For this review, take the finished solid that the model builds, in its own axes (mm). A direction names the side the tool comes from. Coordinates: 2 decimals unless noted, no trailing zeros. Loops run counter-clockwise (first coordinate to the right, second up) from the corner with the lowest first, then second, coordinate; pieces in that order, holes last. Notation, with made-up numbers: (-26.5, 80.25) -> (-14.5, 80.25) arc R3 cw to (-14.5, 84.25) -> close; hole circle Ø7 at (80.25, 86.25). An arc over 180 degrees is marked (long way). Use a Markdown table: item, result.
from build123d import *

# Parameters (mm, degrees)
SKETCH1_R           = 10.16
BOSS_EXTRUDE1_DEPTH = 88.9
FILLET1_R           = 2.54
SKETCH3_W           = 15.24
SKETCH3_H           = 10.16
BOSS_EXTRUDE2_DEPTH = 30.48
FILLET2_R           = 7.62
CUT_EXTRUDE1_REACH  = 97.208
SKETCH4_R           = 5.08
FILLET3_R           = 2.54


with BuildPart() as part:
    # Sketch1 → Boss-Extrude1 (new, symmetric)
    with BuildSketch(Plane.XY):
        Circle(SKETCH1_R)
    extrude(amount=BOSS_EXTRUDE1_DEPTH, both=True)

    # Fillet1
    fillet1_edges = [part.edges().sort_by_distance(p)[0] for p in [
        (-10.16, 0, -88.9),
        (-10.16, 0, 88.9),
    ]]
    fillet(fillet1_edges, radius=FILLET1_R)

    # Sketch3 → Boss-Extrude2 (add)
    with BuildSketch(Plane(origin=(0, 0, 0), x_dir=(0, 0, -1), z_dir=(1, 0, 0))):
        with Locations((73.66, 0)):
            Rectangle(SKETCH3_W, SKETCH3_H)
    extrude(amount=BOSS_EXTRUDE2_DEPTH)

    # Fillet2
    fillet2_edges = [part.edges().sort_by_distance(p)[0] for p in [
        (30.48, 0, -81.28),
        (30.48, 0, -66.04),
    ]]
    fillet(fillet2_edges, radius=FILLET2_R - 0.0001)  # a hair under: the kernel refuses the full size

    # Sketch4 → Cut-Extrude1 (cut, up to next)
    with BuildSketch(Plane(origin=(0, 5.08, 0), x_dir=(1, 0, 0), z_dir=(0, 1, 0)), mode=Mode.PRIVATE) as cut_extrude1_sk1:
        with Locations(Location((22.86, 73.66, 0), (0, 0, 270))):
            Circle(SKETCH4_R)
    cut_extrude1_tool1 = extrude(cut_extrude1_sk1.sketch, amount=-CUT_EXTRUDE1_REACH, mode=Mode.PRIVATE) & part.part
    add(cut_extrude1_tool1.solids().sort_by_distance((22.86, 5.08, -73.66))[0], mode=Mode.SUBTRACT)

    # Fillet3
    fillet3_edges = [part.edges().sort_by_distance(p)[0] for p in [
        (8.798818102, -5.08, -73.66),
        (9.813806395, 2.629601498, -66.04),
        (8.798818102, 5.08, -73.66),
        (9.813806395, -2.629601498, -81.28),
    ]]
    fillet(fillet3_edges, radius=FILLET3_R)


solid = part.part
(1) For faces 1 (the face through (0, 0, 88.9)), 2 (the face through (17.9, 5.08, -71.8)), 3 (the face through (17.9, -5.08, -71.8)), list the 3-axis set-ups (+Z, -Z, +X, -X, +Y, -Y) from which the entire face can be reached by the end or side of a thin tool; tool diameter is ignored.
Found:
| item | result |
|---|---|
| face 1 | +Z, +X, -X, +Y, -Y |
| face 2 | +Z, -Z, +X, +Y |
| face 3 | +Z, -Z, +X, -Y |
(2) For line 1 along X through (y, z) = (0.5, -73.66); line 2 along X through (y, z) = (1.5, -73.66); line 3 along X through (y, z) = (-0.5, 41), list the stretches that pass through material, from the lowest coordinate up.
Found:
| item | result |
|---|---|
| line 1 | x = -10.15 to 17.78, 27.94 to 30.48 |
| line 2 | x = -10.05 to 17.78, 27.94 to 30.48 |
| line 3 | x = -10.15 to 10.15 |
(3) Take a section at B-B on z = 66.5. Write out the cut boundary in (x, y), plus the area to 3 significant figures.
Found:
| item | result |
|---|---|
| outline | circle Ø20.32 at (0, 0) |
| area | 324 mm^2 |
(4) For pin 1 Ø13 at (x, z) = (23, -75) entering from +Y; pin 2 Ø3 at (x, y) = (17.5, 2.5) entering from -Z; pin 3 Ø12 at (x, y) = (17, 0) entering from -Z, all flat-tipped, find the tip position at first contact; note any pin that passes through.
Found:
| item | result |
|---|---|
| pin 1 | stops at y = 5.08 |
| pin 2 | stops at z = -81.28 |
| pin 3 | stops at z = -81.93 |
(5) Mouldability with a two-part tool opening along Z and no side actions: class faces 4 (the face through (19.77, 0.07, -77.69)), 5 (the face through (17, 0, -66.04)), 6 (the face through (28.307, 0.071, -78.989)) as pulls with the +Z half, pulls with the -Z half, needs draft (parallel to the pull), parting line crosses it, or undercut.
Found:
| item | result |
|---|---|
| face 4 | undercut |
| face 5 | pulls with the +Z half |
| face 6 | pulls with the -Z half |
